Geometry check sheet. Reference: the model listing, model coordinates, mm. Coordinates: 2 decimals unless noted, no trailing zeros. Write each loop counter-clockwise with the first axis right and the second up, starting at its lowest first coordinate (ties: lowest second). Pieces come first, ordered by that corner, then holes. Notation, with made-up numbers: (26, -2.75) -> (52, -2.75) arc R22 cw to (52, 29.25) -> close; hole circle Ø11 at (8.5, 73.25). An arc over 180 degrees is marked (long way). One line per question, with ' | ' between items.
```python
from build123d import *

# Parameters (mm, degrees)
SKETCH1_W                    = 131.490901353
SKETCH1_H                    = 105.083375897
SKETCH1_R                    = 1.9812
BASE_PLATE_DEPTH             = 6.35
SKETCH2_R                    = 1.6
SKETCH2_R_2                  = 1.540770003
ARDUINO_MOUNTING_HOLES_DEPTH = 6.35
SKETCH3_W                    = 41.532415145
SKETCH3_H                    = 77.800157949
CABLE_OPENING_DEPTH          = 6.35
SKETCH4_W                    = 74.20112143
SKETCH4_H                    = 5.509329328
SKETCH4_W_2                  = 72.501511829
SKETCH4_H_2                  = 5.116757241
SKETCH4_W_3                  = 5.306940646
SKETCH4_H_3                  = 50.003346063
CUT_EXTRUDE3_DEPTH           = 6.35


with BuildPart() as part:
    # Sketch1 → Base_Plate (new body)
    with BuildSketch(Plane.XY.offset(1332.023843603)):
        with Locations((483.923899553, 868.728663849)):
            Rectangle(SKETCH1_W, SKETCH1_H)
        with Locations((423.356809583, 913.820206664)):
            Circle(SKETCH1_R, mode=Mode.SUBTRACT)
        with Locations((544.362409583, 913.820206664)):
            Circle(SKETCH1_R, mode=Mode.SUBTRACT)
        with Locations((544.362409583, 823.802606664)):
            Circle(SKETCH1_R, mode=Mode.SUBTRACT)
        with Locations((423.356809583, 823.802606664)):
            Circle(SKETCH1_R, mode=Mode.SUBTRACT)
    extrude(amount=BASE_PLATE_DEPTH)

    # Sketch2 → Arduino_Mounting_Holes (cut)
    with BuildSketch(Plane.XY.offset(1338.373843603)):
        with Locations((486.149027751, 893.958307234)):
            Circle(SKETCH2_R)
        with Locations((537.005692703, 879.063667595)):
            Circle(SKETCH2_R_2)
        with Locations((537.262931981, 851.150350094)):
            Circle(SKETCH2_R)
        with Locations((485.231408993, 845.690321199)):
            Circle(SKETCH2_R)
    extrude(amount=-ARDUINO_MOUNTING_HOLES_DEPTH, mode=Mode.SUBTRACT)

    # Sketch3 → Cable_Opening (cut)
    with BuildSketch(Plane.XY.offset(1338.373843603)):
        with Locations((445.669830045, 869.267134618)):
            Rectangle(SKETCH3_W, SKETCH3_H)
    extrude(amount=-CABLE_OPENING_DEPTH, mode=Mode.SUBTRACT)

    # Sketch4 → Cut-Extrude3 (cut)
    with BuildSketch(Plane.XY.offset(1338.373843603)):
        with Locations((504.759181332, 918.515687133)):
            Rectangle(SKETCH4_W, SKETCH4_H)
        with Locations((503.90881977, 818.745354521)):
            Rectangle(SKETCH4_W_2, SKETCH4_H_2)
        with Locations((547.015879906, 866.253246095)):
            Rectangle(SKETCH4_W_3, SKETCH4_H_3)
    extrude(amount=-CUT_EXTRUDE3_DEPTH, mode=Mode.SUBTRACT)


solid = part.part
```
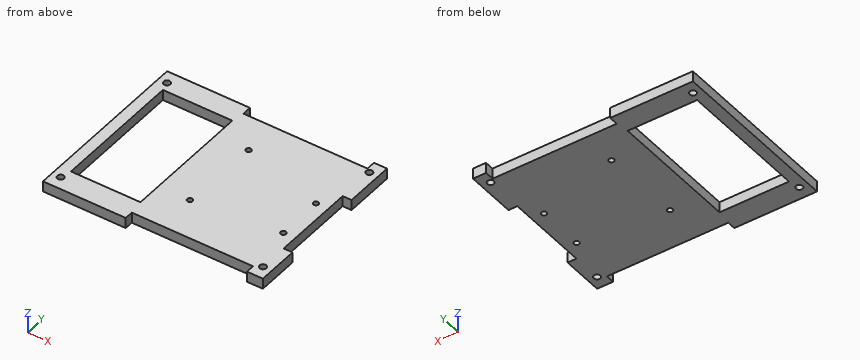
(1) Depth check by flat-ended pin: P1, Ø3, axis at y = 871.5, z = 1336.5, coming from the +X side; P2, Ø3, axis at x = 530, z = 1336, coming from the -Y side; P3, Ø2.5, axis at x = 537.01, y = 879.06, coming from the +Z side; P4, Ø6.5, axis at x = 544.36, y = 913.82, coming from the -Z side. Enter the tip coordinate at first touch or a pass-through.
Answers below:
P1: stops at x = 544.36 | P2: stops at y = 821.3 | P3: passes through | P4: stops at z = 1332.02
(2) Cross-section at B-B (y = 899). Record the cut outline in (x, z), plus the area to 3 significant figures.
Answers below:
outline: (418.18, 1332.02) -> (424.9, 1332.02) -> (424.9, 1338.37) -> (418.18, 1338.37) -> close; (466.44, 1332.02) -> (549.67, 1332.02) -> (549.67, 1338.37) -> (466.44, 1338.37) -> close | area: 571 mm²
(3) Cross-section at D-D (x = 534). Record the cut outline in (y, z), plus the area to 3 significant figures.
Answers below:
outline: (821.3, 1332.02) -> (915.76, 1332.02) -> (915.76, 1338.37) -> (821.3, 1338.37) -> close | area: 600 mm²
(4) Material ranges on line 1 (X direction, y = 823.5, z = 1333.25); line 2 (Y direction, x = 437, z = 1333); line 3 (X direction, y = 847.5, z = 1337.75), recorded low to high.
Answers below:
line 1: x = 418.18 to 421.4, 425.31 to 542.4, 546.32 to 549.67 | line 2: y = 816.19 to 830.37, 908.17 to 921.27 | line 3: x = 418.18 to 424.9, 466.44 to 544.36
(5) Cross-section at A-A (x = 452). Record the cut outline in (y, z), plus the area to 3 significant figures.
Answers below:
outline: (816.19, 1332.02) -> (830.37, 1332.02) -> (830.37, 1338.37) -> (816.19, 1338.37) -> close; (908.17, 1332.02) -> (921.27, 1332.02) -> (921.27, 1338.37) -> (908.17, 1338.37) -> close | area: 173 mm²
(6) Cross-section at C-C (z = 1337). Count the separate pieces of the cut face and the enclosed holes in it, plus the area to 3 significant figures.
Answers below:
separate pieces: 1 | enclosed holes: 9 | area: 9,460 mm²
